CAD build for the part. Positions are in the model's coordinates, mm. Coordinates: 2 decimals unless noted, no trailing zeros. Write each loop counter-clockwise with the first axis right and the second up, starting at its lowest first coordinate (ties: lowest second). Pieces come first, ordered by that corner, then holes. Notation, with made-up numbers: (65, -38.5) - (115, -38.5) arc R24 ccw to (115, -3.5) - close; hole circle Ø4 at (44, 41.5). An arc over 180 degrees is marked (long way). Answer in a Markdown table with one row per item. Add a question column.
Q1. Band-saw the part on C-C (z = 0). List the corners of the cut face in (x, y).
Q2. Band-saw the part on A-A (y = 0). List the corners of the cut face in (x, z).
Q3. Band-saw the part on B-B (x = 1.05). List the corners of the cut face in (y, z).
Q4. Drill centre lines: line 1 along Y through (x, z) = (2.2, 2.5); line 2 along Y through (x, z) = (2.4, 45). Where is each one in solid material? Low to high. Write a range as from..to.
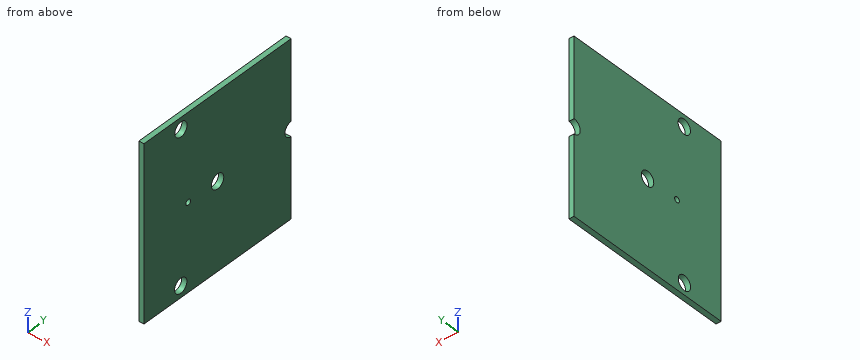
```python
from build123d import *

# Parameters (mm, degrees)
SKETCH2_W           = 100
SKETCH2_H           = 100
SKETCH2_R           = 4.2
BOSS_EXTRUDE1_DEPTH = 3
SKETCH3_R           = 4.2
CUT_EXTRUDE1_DEPTH  = 10
SKETCH4_R           = 1.6
CUT_EXTRUDE2_DEPTH  = 10


with BuildPart() as part:
    # Sketch2 → Boss-Extrude1 (new body)
    with BuildSketch(Plane(origin=(0, 0, 0), x_dir=(0, 0, -1), z_dir=(1, 0, 0))):
        Rectangle(SKETCH2_W, SKETCH2_H)
        Circle(SKETCH2_R, mode=Mode.SUBTRACT)
    extrude(amount=BOSS_EXTRUDE1_DEPTH)

    # Sketch3 → Cut-Extrude1 (cut)
    with BuildSketch(Plane.ZY):
        with Locations((43.336976945, -24.938051834)):
            Circle(SKETCH3_R)
        with Locations((-43.265474881, -25.061897041)):
            Circle(SKETCH3_R)
        with Locations((-0.071502064, 49.999948875)):
            Circle(SKETCH3_R)
    extrude(amount=-CUT_EXTRUDE1_DEPTH, mode=Mode.SUBTRACT)

    # Sketch4 → Cut-Extrude2 (cut)
    with BuildSketch(Plane.ZY):
        with Locations((0, -20)):
            Circle(SKETCH4_R)
    extrude(amount=-CUT_EXTRUDE2_DEPTH, mode=Mode.SUBTRACT)


solid = part.part
```
Checked values:
| question | item | result |
|---|---|---|
| 1 | outline | (0, -50) - (3, -50) - (3, -21.6) - (0, -21.6) - close; (0, -18.4) - (3, -18.4) - (3, -4.2) - (0, -4.2) - close; (0, 4.2) - (3, 4.2) - (3, 45.8) - (0, 45.8) - close |
| 2 | outline | (0, -50) - (3, -50) - (3, -4.2) - (0, -4.2) - close; (0, 4.2) - (3, 4.2) - (3, 50) - (0, 50) - close |
| 3 | outline | (-50, -50) - (50, -50) - (50, -4.27) arc R4.2 cw to (50, 4.13) - (50, 50) - (-50, 50) - close; hole circle Ø8.4 at (-25.06, -43.27); hole circle Ø8.4 at (-24.94, 43.34); hole circle Ø3.2 at (-20, 0); hole circle Ø8.4 at (0, 0) |
| 4 | line 1 | y = -50..-3.37, 3.37..46.68 |
| 4 | line 2 | y = -50..-28.79, -21.08..50 |
